Source: CAD feature listing. Evaluate the final solid. Frame: model axes, mm. A direction names the side the tool comes from. Give positions to 0.01 mm unless a question says otherwise; leave off trailing zeros. Order: outer loops, then holes, each group sorted by start corner. A loop starts at its lowest first (then second) coordinate and runs counter-clockwise, first axis right, second up.
1) First-contact query: P1, Ø6, axis at x = 114.3, z = -4.93, coming from the +Y side (3 decimals); P2, Ø3, axis at x = 146, y = 3, coming from the -Z side; P3, Ø5, axis at y = 6.5, z = -9, coming from the +X side; P4, Ø3, axis at y = 4, z = -8, coming from the -X side. Flat tips, straight axial feed; report the tip coordinate or a pass-through.
2) Section A-A, the plane y = 2.25. Return loops of the section in (x, z) (3 decimals), plus the area to 3 significant figures.
3) Access query for faces 1 (the face through (144, 5, 7.62)), 2 (the face through (-139.7, 5, -10)), 3 (the face through (-144, 5, 7.62)). Directions: +Z, -Z, +X, -X, +Y, -Y. A direction counts if a zero-diameter tool reaches every point of the face in a straight line with its end or side. Return the directions, or none.
4) Material intervals for line 1 (Z direction, x = -114.3, y = 3.5); line 2 (X direction, y = 1, z = -7.5); line 3 (Z direction, x = -76, y = 1.25), sorted ascending.
5) Draft query along Z for faces 4 (the face through (-139.7, 5, 11)), 5 (the face through (-116.53, 4.7, -4.23)), 6 (the face through (-2, 5, 15.24)). Return one class per face: released by +Z, released by -Z, zero draft, split by the parting line, or undercut.
```python
from build123d import *

# Parameters (mm, degrees)
SKETCH1_W           = 279.4
SKETCH1_H           = 30.48
BOSS_EXTRUDE1_DEPTH = 9.525
SKETCH2_W           = 12.7
SKETCH2_H           = 9.525
BOSS_EXTRUDE2_DEPTH = 9.525
SKETCH3_R           = 2.3368
CUT_EXTRUDE1_DEPTH  = 10.525


with BuildPart() as part:
    # Sketch1 → Boss-Extrude1 (new body)
    with BuildSketch(Plane(origin=(0, 0, 0), x_dir=(1, 0, 0), z_dir=(0, 1, 0))):
        Rectangle(SKETCH1_W, SKETCH1_H)
    extrude(amount=BOSS_EXTRUDE1_DEPTH)

    # Sketch2 → Boss-Extrude2 (add)
    with BuildSketch(Plane(origin=(139.7, 0, 0), x_dir=(0, 0, -1), z_dir=(1, 0, 0))):
        with Locations((-1.27, 4.7625)):
            Rectangle(SKETCH2_W, SKETCH2_H)
    boss_extrude2 = extrude(amount=BOSS_EXTRUDE2_DEPTH)

    # Mirror1: Boss-Extrude2 across plane
    add(boss_extrude2.mirror(Plane(origin=(0, 0, 0), x_dir=(0, 0, 1), z_dir=(1, 0, 0))))

    # Sketch3 → Cut-Extrude1 (cut, through all)
    with BuildSketch(Plane.XZ):
        with Locations((114.3, -4.9276)):
            Circle(SKETCH3_R)
        with Locations((77.7748, -4.9276)):
            Circle(SKETCH3_R)
        with Locations((96.0374, -4.9276)):
            Circle(SKETCH3_R)
    cut_extrude1 = extrude(amount=-CUT_EXTRUDE1_DEPTH, mode=Mode.SUBTRACT)

    # Mirror2: Cut-Extrude1 across plane
    add(cut_extrude1.mirror(Plane(origin=(0, 0, 0), x_dir=(0, 0, 1), z_dir=(1, 0, 0))), mode=Mode.SUBTRACT)


solid = part.part
```
From the geometry:
1. P1: stops at y = 9.525
1. P2: stops at z = -5.08
1. P3: stops at x = 139.7
1. P4: stops at x = -139.7
2. outline: (-149.225, -5.08) - (-139.7, -5.08) - (-139.7, -15.24) - (139.7, -15.24) - (139.7, -5.08) - (149.225, -5.08) - (149.225, 7.62) - (139.7, 7.62) - (139.7, 15.24) - (-139.7, 15.24) - (-139.7, 7.62) - (-149.225, 7.62) - close; hole circle Ø4.674 at (-114.3, -4.928); hole circle Ø4.674 at (-96.037, -4.928); hole circle Ø4.674 at (-77.775, -4.928); hole circle Ø4.674 at (77.775, -4.928); hole circle Ø4.674 at (96.037, -4.928); hole circle Ø4.674 at (114.3, -4.928)
2. area: 8,660 mm2
3. face 1: +Z, +X, +Y, -Y
3. face 2: -Z, -X, +Y, -Y
3. face 3: +Z, -X, +Y, -Y
4. line 1: z = -15.24 to -7.26, -2.59 to 15.24
4. line 2: x = -139.7 to 139.7
4. line 3: z = -15.24 to -6.45, -3.41 to 15.24
5. face 4: zero draft
5. face 5: undercut
5. face 6: released by +Z
